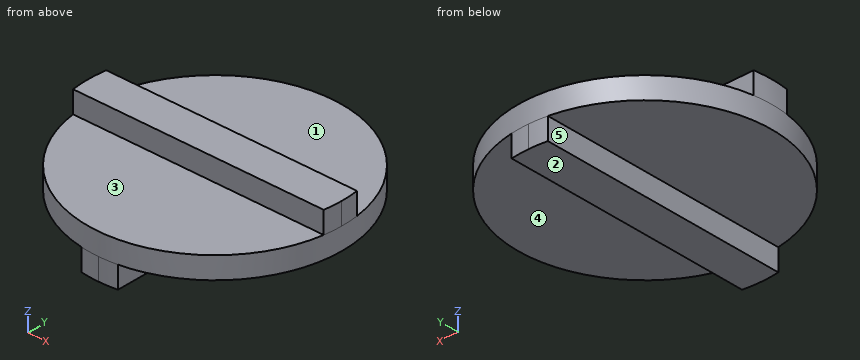
```python
from build123d import *

# Parameters (mm, degrees)
SKETCH1_R           = 17.5
BOSS_EXTRUDE1_DEPTH = 3
BOSS_EXTRUDE2_DEPTH = 3
BOSS_EXTRUDE3_DEPTH = 3


with BuildPart() as part:
    # Sketch1 → Boss-Extrude1 (new body)
    with BuildSketch(Plane.XY):
        Circle(SKETCH1_R)
    extrude(amount=BOSS_EXTRUDE1_DEPTH)

    # Sketch2 → Boss-Extrude2 (add)
    with BuildSketch(Plane.XY.offset(3)):
        with BuildLine():
            Line((0, 2.5), (-17.320508076, 2.5))
            ThreePointArc((-17.320508076, 2.5), (-17.5, 0), (-17.320508076, -2.5))
            Line((-17.320508076, -2.5), (0, -2.5))
            Line((0, -2.5), (0, 2.5))
        make_face()
        with BuildLine():
            Line((17.320508076, 2.5), (0, 2.5))
            Line((0, 2.5), (0, -2.5))
            Line((0, -2.5), (17.320508076, -2.5))
            ThreePointArc((17.320508076, -2.5), (17.45506934, -1.253217594), (17.5, 0))
            ThreePointArc((17.5, 0), (17.45506934, 1.253217594), (17.320508076, 2.5))
        make_face()
    extrude(amount=BOSS_EXTRUDE2_DEPTH)

    # Sketch3 → Boss-Extrude3 (add)
    with BuildSketch(Plane(origin=(0, 0, 0), x_dir=(-1, 0, 0), z_dir=(0, 0, -1))):
        with BuildLine():
            ThreePointArc((0, 17.5), (-1.253217594, 17.45506934), (-2.5, 17.320508076))
            Line((-2.5, 17.320508076), (-2.5, -17.320508076))
            ThreePointArc((-2.5, -17.320508076), (-1.253217594, -17.45506934), (0, -17.5))
            Line((0, -17.5), (0, 17.5))
        make_face()
        with BuildLine():
            ThreePointArc((2.5, 17.320508076), (1.253217594, 17.45506934), (0, 17.5))
            Line((0, 17.5), (0, -17.5))
            ThreePointArc((0, -17.5), (1.253217594, -17.45506934), (2.5, -17.320508076))
            Line((2.5, -17.320508076), (2.5, 17.320508076))
        make_face()
    extrude(amount=BOSS_EXTRUDE3_DEPTH)


solid = part.part
```
Can you work these out from the model? Positions are in its coordinate system, mm. Face numbers are marked on the shaded views. A direction names the side the tool comes from. Coordinates: 2 decimals unless noted, no trailing zeros. Order: outer loops, then holes, each group sorted by start corner. A loop starts at its lowest first (then second) coordinate and runs counter-clockwise, first axis right, second up. Notation, with made-up numbers: (68, 62.5) - (75, 62.5) arc R12 cw to (75, 75.5) - close; hole circle Ø8 at (40, -2). An arc over 180 degrees is marked (long way). Answer in a Markdown table with one row per item.
1. Suppose I cut it at A-A (x = -7). Please give me the cut outline in (y, z).
Reply:
| item | result |
|---|---|
| outline | (-16.04, 0) - (16.04, 0) - (16.04, 3) - (2.5, 3) - (2.5, 6) - (-2.5, 6) - (-2.5, 3) - (-16.04, 3) - close |
2. Suppose I cut it at B-B (z = -2). Please give me the cut outline in (x, y).
Reply:
| item | result |
|---|---|
| outline | (-2.5, -17.32) arc R17.5 ccw to (2.5, -17.32) - (2.5, 17.32) arc R17.5 ccw to (-2.5, 17.32) - close |
3. If I drill on line 1 along X through (y, z) = (11, -1.25); line 2 along Z through (x, y) = (-9, -11.5), over which ranges is the centre line in solid material (lowest first)?
Reply:
| item | result |
|---|---|
| line 1 | x = -2.5 to 2.5 |
| line 2 | z = 0 to 3 |
4. Suppose I cut it at C-C (y = 8). Please give me the cut outline in (x, z), and give its area (3 significant figures).
Reply:
| item | result |
|---|---|
| outline | (-15.56, 0) - (-2.5, 0) - (-2.5, -3) - (2.5, -3) - (2.5, 0) - (15.56, 0) - (15.56, 3) - (-15.56, 3) - close |
| area | 108 mm^2 |
5. For pin 1 (3.5 mm diameter, centred on y = 5.5, z = -1, fed in from -X); pin 2 (1 mm diameter, centred on x = -3, y = 7, fed in from +Z); pin 3 (0.9 mm diameter, centred on x = 2, z = 5, fed in from +Y), each with a flat end and sliding along its axis, tell me the tip position at first contact or that it passes through.
Reply:
| item | result |
|---|---|
| pin 1 | stops at x = -17.02 |
| pin 2 | stops at z = 3 |
| pin 3 | stops at y = 2.5 |
6. Suppose I cut it at D-D (z = 1.5). Please give me the cut outline in (x, y), and give its area (3 significant figures).
Reply:
| item | result |
|---|---|
| outline | circle Ø35 at (0, 0) |
| area | 962 mm^2 |
7. For the marked faces 1, 2, 3, 4 and 5, which set-ups out of +Z, -Z, +X, -X, +Y, -Y let a thin tool reach every point of the face, with its end or its side?
Reply:
| item | result |
|---|---|
| face 1 | +Z, +X, -X, +Y |
| face 2 | -Z, +X, -X, +Y, -Y |
| face 3 | +Z, +X, -X, -Y |
| face 4 | -Z, +X, +Y, -Y |
| face 5 | -Z, -X, +Y, -Y |
